The model under review builds one solid part; all positions refer to its coordinate system, in mm. Round coordinates to 2 decimals unless told otherwise and drop trailing zeros. Order: outer loops, then holes, each group sorted by start corner. A loop starts at its lowest first (then second) coordinate and runs counter-clockwise, first axis right, second up. Notation, with made-up numbers: (20, -7) -> (24, -7) arc R4 ccw to (24, -2) -> close; hole circle Ø9 at (7.25, 3.5). An arc over 180 degrees is marked (long way). Return JSON: item names as keys, results as strings. Group by question number.
Autodesk Inventor part; units mm, degrees
ref_plane "YZ Plane" through (0, 0, 0) normal (1, 0, 0) x (0, 1, 0)
ref_plane "XZ Plane" through (0, 0, 0) normal (0, 1, 0) x (-1, 0, 0)
ref_plane "XY Plane" through (0, 0, 0) normal (0, 0, 1) x (1, 0, 0)
sketch "Sketch1" plane through (0, 0, 0) normal (0, 0, 1) x (1, 0, 0)
  point P0 (0, 0)
sketch "Sketch2" plane through (0, 0, 0) normal (0, 0, 1) x (1, 0, 0)
  point P0 (0, 0)
sketch "Sketch3" plane through (0, 0, 0) normal (0, 0, 1) x (1, 0, 0)
  circle A0 centre (0, 0) radius 38.5
  dimension "d0" = 77
extrude "Extrusion1" add sketch "Sketch3" along normal blind 80
sketch "Sketch4" plane through (0, 0, 80) normal (0, 0, 1) x (1, 0, 0)
  circle A0 centre (0, 0) radius 4
  dimension "d3" = 8
extrude "Extrusion2" cut sketch "Sketch4" against normal blind 15
sketch "Sketch5" plane through (0, 0, 80) normal (0, 0, 1) x (1, 0, 0)
  point P0 (0, 0)
sketch "Sketch6" plane through (0, 0, 0) normal (0, 0, -1) x (-1, 0, 0)
  circle A0 centre (0, 0) radius 4
  circle A1 centre (0, 0) radius 4
  dimension "d6" = 8
extrude "Extrusion3" cut sketch "Sketch6" against normal blind 150
properties part number "roller of 4 cm"
Item 1: Consider section C-C on z = 40. State the section outline as (x, y) points.
Item 2: Consider section D-D on x = -21.5. State the section outline as (y, z) points, plus the area to 3 significant figures.
Item 3: Consider section A-A on y = 0. State the section outline as (x, z) points, plus the area to 3 significant figures.
Item 4: The part is to be moulded in two halves that separate along Y. For faces 1 (the face through (-1, -8, 80)), 2 (the face through (-30.55, 23.43, 39.44)), 3 (the face through (0, 4, 39)), say which applies: +Y half, -Y half, draft (parallel to the pull), parting line (faces both ways), or undercut.
Item 5: Insertion check: pin 1 Ø1.5 at (y, z) = (1.5, 15) entering from +X; pin 2 Ø2 at (x, z) = (16.5, 33.5) entering from +Y; pin 3 Ø2 at (x, y) = (29.5, 28) entering from -Z; pin 4 Ø1 at (x, z) = (7, 32.5) entering from +Y. Each pin has a flat end and moves straight along its axis. Give the tip position at first contact, or say it passes through.
Item 6: Wall thickness on line 1 along Y through (x, z) = (0, 56.5); line 2 along Y through (x, z) = (-3, 22.5); line 3 along Y through (x, z) = (15, 55): over which ranges is each line inside the solid? List them lowest first.
Values:
{
 "1": {"outline": "circle Ø77 at (0, 0); hole circle Ø8 at (0, 0)"},
 "2": {"outline": "(-31.94, 0) -> (31.94, 0) -> (31.94, 80) -> (-31.94, 80) -> close", "area": "5,110 mm^2"},
 "3": {"outline": "(-38.5, 0) -> (-4, 0) -> (-4, 80) -> (-38.5, 80) -> close; (4, 0) -> (38.5, 0) -> (38.5, 80) -> (4, 80) -> close", "area": "5,520 mm^2"},
 "4": {"face 1": "draft", "face 2": "parting line", "face 3": "undercut"},
 "5": {"pin 1": "x = 38.49", "pin 2": "y = 35.24", "pin 3": "through", "pin 4": "y = 37.95"},
 "6": {"line 1": "-38.5 to -4, 4 to 38.5", "line 2": "-38.38 to -2.65, 2.65 to 38.38", "line 3": "-35.46 to 35.46"}
}
